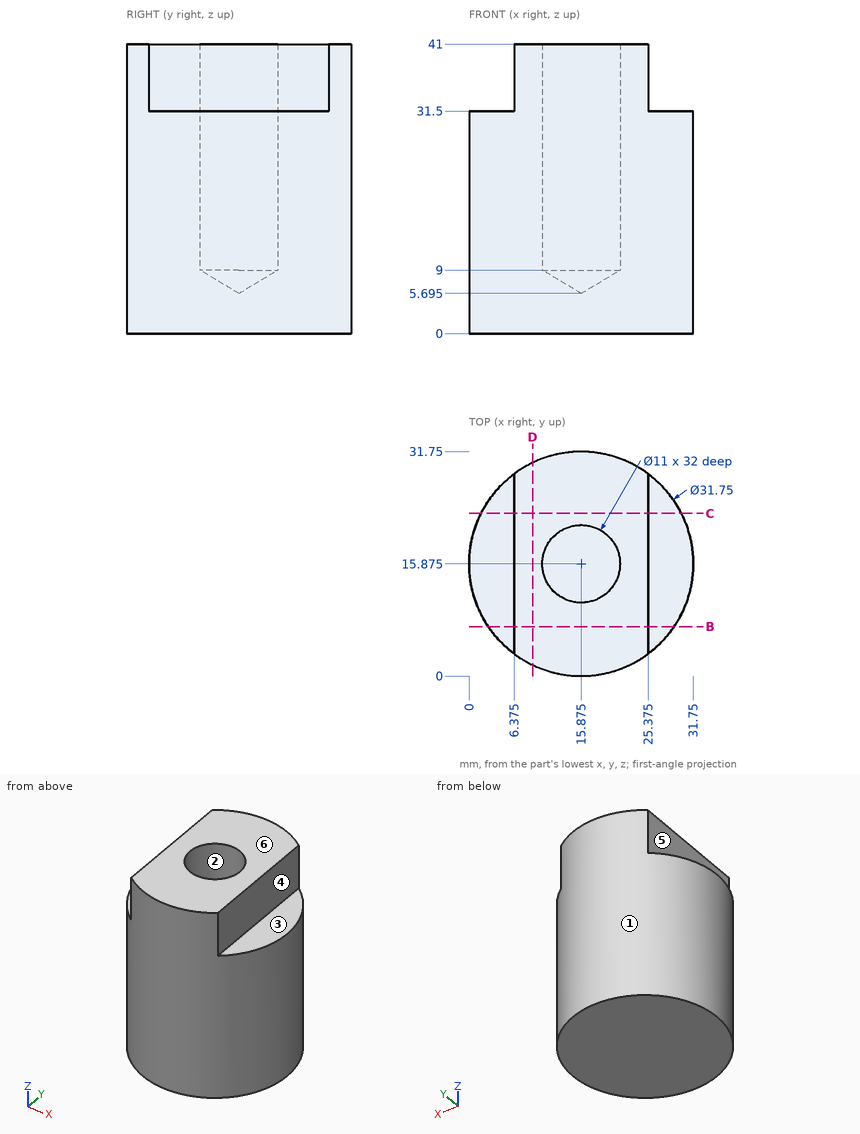
Geometry: see drawing. Coordinates: mm, zero at the bounding-box minimum. A direction names the side the tool comes from. Coordinates: 2 decimals unless noted, no trailing zeros. Order: outer loops, then holes, each group sorted by start corner. A loop starts at its lowest first (then second) coordinate and runs counter-clockwise, first axis right, second up. Notation, with made-up numbers: (-15, 83) - (44, 83) arc R30 ccw to (44, 122) - close; hole circle Ø9 at (78.5, 55.25). An arc over 180 degrees is marked (long way). Return JSON: item names as keys, results as strings.
Q1. Cut plane D-D (x = 9). Return loops of the section in (y, z).
The answers:
{"outline": "(1.57, 0) - (30.18, 0) - (30.18, 41) - (1.57, 41) - close"}
Q2. Cut plane C-C (y = 23). Return loops of the section in (x, z) (1 decimal).
The answers:
{"outline": "(1.7, 0) - (30.1, 0) - (30.1, 31.5) - (25.4, 31.5) - (25.4, 41) - (6.4, 41) - (6.4, 31.5) - (1.7, 31.5) - close"}
Q3. Draft query along Y for the marked faces 1, 2 and 3. Return one class per face: +Y half, -Y half, draft (parallel to the pull), parting line (faces both ways), or undercut.
The answers:
{"face 1": "parting line", "face 2": "undercut", "face 3": "draft"}
Q4. Access query for the marked faces 4, 5 and 6. Directions: +Z, -Z, +X, -X, +Y, -Y. A direction counts if a zero-diameter tool reaches every point of the face in a straight line with its end or side. Return the directions, or none.
The answers:
{"face 4": "+Z, +X, +Y, -Y", "face 5": "+Z, -X, +Y, -Y", "face 6": "+Z, +X, -X, +Y, -Y"}
Q5. Cut plane B-B (y = 7). Return loops of the section in (x, z) (1 decimal), then the cut area to 3 significant figures.
The answers:
{"outline": "(2.7, 0) - (29, 0) - (29, 31.5) - (25.4, 31.5) - (25.4, 41) - (6.4, 41) - (6.4, 31.5) - (2.7, 31.5) - close", "area": "1,010 mm2"}
Q6. First-contact query: pin 1 (3 mm diameter, centred on y = 26.5, z = 29.5, fed in from +X) (1 decimal); pin 2 (10 mm diameter, centred on x = 15.875, y = 15.875, fed in from +Z); pin 3 (10 mm diameter, centred on x = 9, z = 34.5, fed in from -Y). Flat tips, straight axial feed; report the tip coordinate or a pass-through.
The answers:
{"pin 1": "stops at x = 28.9", "pin 2": "stops at z = 8.7", "pin 3": "stops at y = 0.11"}
Q7. Ray query, probe 1 along X at (y, z) = (16, 25); probe 2 along X at (y, z) = (6, 34) (1 decimal); probe 3 along Y at (x, z) = (12.5, 21.5). Return the intervals inside material, ascending.
The answers:
{"probe 1": "x = 0 to 10.38, 21.37 to 31.75", "probe 2": "x = 6.4 to 25.4", "probe 3": "y = 0.36 to 11.53, 20.22 to 31.39"}
